Here's how the part is built. I have some questions about the finished solid (model axes, mm). A direction names the side the tool comes from. Round coordinates to 2 decimals unless told otherwise and drop trailing zeros. Write each loop counter-clockwise with the first axis right and the second up, starting at its lowest first coordinate (ties: lowest second). Pieces come first, ordered by that corner, then holes. Notation, with made-up numbers: (-3, -35.75) -> (1, -35.75) arc R24 cw to (1, -0.75) -> close; hole circle Ø11 at (24, -9.75). An arc over 180 degrees is marked (long way). Put each result on its own line as item: value. Start each with the question number.
1) If I drill on line 1 along Y through (x, z) = (8, 8); line 2 along X through (y, z) = (-8.5, 49), over which ranges is the centre line in solid material (lowest first)? Write a range as [from, to].
2) I want a section at C-C, the plane y = -1.25. List the corners of the cut face in (x, z) for me.
3) I want a section at A-A, the plane y = 5.25. List the corners of the cut face in (x, z) for me, then the cut area to 3 significant figures.
4) I want a section at D-D, the plane x = 5. List the corners of the cut face in (y, z) for me.
5) We'd pull the mould along Y, two halves only. Please class faces 1 (the flat face through (2, 3.78, 26)), 2 (the flat face through (6, -10, 26)), 3 (the flat face through (-6.08, 8, 26)): released by +Y, released by -Y, zero draft, split by the parting line, or undercut.
6) I want a section at B-B, the plane x = -1. List the corners of the cut face in (y, z) for me, then the cut area to 3 significant figures.
7) Will these pins go through, and if not, where does the flat tip stop? P1, Ø3, axis at x = -1.5, z = 22.5, coming from the -Y side; P2, Ø6, axis at x = 6.5, y = 3.5, coming from the -Z side; P3, Ø0.8, axis at y = -1.5, z = 16.5, coming from the -X side; P4, Ø3, axis at x = 1.5, z = 28, coming from the +Y side.
8) Which directions (+Z, -Z, +X, -X, +Y, -Y) give clear straight access to the entire face, cutting with the end or side of a thin tool? Please do faces 4 (the flat face through (-2, -3.78, 26)), 5 (the flat face through (5, -8.2, 26)), 6 (the flat face through (-9, -3.3, 26)).
from build123d import *

# Parameters (mm, degrees)
SKETCH1_R           = 2.05
BOSS_EXTRUDE1_DEPTH = 51.85
FILLET1_R           = 0.5


with BuildPart() as part:
    # Sketch1 → Boss-Extrude1 (new body)
    with BuildSketch(Plane.XY):
        Polygon((-3.3, 10), (-3.3, 8.2), (-6.08, 8.2), (-6.08, 6.928528137), (-2.931471863, 3.78), (-0.34, 3.78), (0, 3.66), (0.34, 3.78), (2.931471863, 3.78), (6.08, 6.928528137), (6.08, 8.2), (3.3, 8.2), (3.3, 10), (10, 10), (10, 3.3), (8.2, 3.3), (8.2, 6.08), (6.928528137, 6.08), (3.78, 2.931471863), (3.78, 0.34), (3.66, 0), (3.78, -0.34), (3.78, -2.931471863), (6.928528137, -6.08), (8.2, -6.08), (8.2, -3.3), (10, -3.3), (10, -10), (3.3, -10), (3.3, -8.2), (6.08, -8.2), (6.08, -6.928528137), (2.931471863, -3.78), (0.34, -3.78), (0, -3.66), (-0.34, -3.78), (-2.931471863, -3.78), (-6.08, -6.928528137), (-6.08, -8.2), (-3.3, -8.2), (-3.3, -10), (-10, -10), (-10, -3.3), (-8.2, -3.3), (-8.2, -6.08), (-6.928528137, -6.08), (-3.78, -2.931471863), (-3.78, -0.34), (-3.66, 0), (-3.78, 0.34), (-3.78, 2.931471863), (-6.928528137, 6.08), (-8.2, 6.08), (-8.2, 3.3), (-10, 3.3), (-10, 10), align=None)
        with Locations(Location((0, 0, 0), (0, 0, 180))):
            Circle(SKETCH1_R, mode=Mode.SUBTRACT)
    extrude(amount=BOSS_EXTRUDE1_DEPTH)

    # Fillet1
    fillet1_edges = [part.edges().sort_by_distance(p)[0] for p in [
        (10, 10, 25.925),
        (10, -10, 25.925),
        (-10, -10, 25.925),
        (-10, 10, 25.925),
    ]]
    fillet(fillet1_edges, radius=FILLET1_R)


solid = part.part
Findings:
1. line 1: y = [-10, -6.08], [6.08, 10]
1. line 2: x = [-10, -3.3], [3.3, 10]
2. outline: (-3.78, 0) -> (-1.62, 0) -> (-1.62, 51.85) -> (-3.78, 51.85) -> close; (1.62, 0) -> (3.78, 0) -> (3.78, 51.85) -> (1.62, 51.85) -> close
3. outline: (-10, 0) -> (-8.2, 0) -> (-8.2, 51.85) -> (-10, 51.85) -> close; (-6.1, 0) -> (-4.4, 0) -> (-4.4, 51.85) -> (-6.1, 51.85) -> close; (4.4, 0) -> (6.1, 0) -> (6.1, 51.85) -> (4.4, 51.85) -> close; (8.2, 0) -> (10, 0) -> (10, 51.85) -> (8.2, 51.85) -> close
3. area: 363 mm2
4. outline: (-10, 0) -> (-8.2, 0) -> (-8.2, 51.85) -> (-10, 51.85) -> close; (-5.85, 0) -> (-4.15, 0) -> (-4.15, 51.85) -> (-5.85, 51.85) -> close; (4.15, 0) -> (5.85, 0) -> (5.85, 51.85) -> (4.15, 51.85) -> close; (8.2, 0) -> (10, 0) -> (10, 51.85) -> (8.2, 51.85) -> close
5. face 1: released by +Y
5. face 2: released by -Y
5. face 3: undercut
6. outline: (-3.78, 0) -> (-1.79, 0) -> (-1.79, 51.85) -> (-3.78, 51.85) -> close; (1.79, 0) -> (3.78, 0) -> (3.78, 51.85) -> (1.79, 51.85) -> close
6. area: 206 mm2
7. P1: stops at y = -3.85
7. P2: stops at z = 0
7. P3: stops at x = -3.78
7. P4: stops at y = 3.85
8. face 4: +Z, -Z, -Y
8. face 5: +Z, -Z
8. face 6: +Z, -Z, -X
